from build123d import *

# Parameters (mm, degrees)
BENCH_FRAME_EXTRUDE_DEPTH    = 3
CURVED_PANEL_CLEARANCE_DEPTH = 4
POD_FOOT_CLEARANCE_SKETCH_R  = 1.7
POD_FOOT_THROUGH_HOLES_DEPTH = 4
FOOT_COUNTERBORE_SKETCH_R    = 3.6
FOOT_COUNTERBORES_DEPTH      = 2.9


with BuildPart() as part:
    # Bench Frame Sketch → Bench Frame Extrude (new, symmetric)
    with BuildSketch(Plane.XY):
        Polygon((-70, -98), (118, -98), (118, 98), (-70, 98), (-70, 83), (62, 83), (62, -83), (-70, -83), align=None)
    extrude(amount=BENCH_FRAME_EXTRUDE_DEPTH, both=True)

    # Curved Panel Clearance Sketch → Curved Panel Clearance (cut, symmetric)
    with BuildSketch(Plane.XY):
        with BuildLine():
            Line((-51.777652934, 90.5), (-45.159619167, 90.5))
            ThreePointArc((-45.159619167, 90.5), (-65.5, 0), (-45.159619167, -90.5))
            Line((-45.159619167, -90.5), (-51.777652934, -90.5))
            ThreePointArc((-51.777652934, -90.5), (-71.5, 0), (-51.777652934, 90.5))
        make_face()
    extrude(amount=CURVED_PANEL_CLEARANCE_DEPTH, both=True, mode=Mode.SUBTRACT)

    # Pod Foot Clearance Sketch → Pod Foot Through Holes (cut, symmetric)
    with BuildSketch(Plane.XY):
        with Locations((-14, -87.5)):
            Circle(POD_FOOT_CLEARANCE_SKETCH_R)
        with Locations((16, -87.5)):
            Circle(POD_FOOT_CLEARANCE_SKETCH_R)
        with Locations((-14, 87.5)):
            Circle(POD_FOOT_CLEARANCE_SKETCH_R)
        with Locations((16, 87.5)):
            Circle(POD_FOOT_CLEARANCE_SKETCH_R)
        with Locations((40.25, 87.5)):
            Circle(POD_FOOT_CLEARANCE_SKETCH_R)
        with Locations((-40.5, 87.5)):
            Circle(POD_FOOT_CLEARANCE_SKETCH_R)
        with Locations((86, 22)):
            Circle(POD_FOOT_CLEARANCE_SKETCH_R)
        with Locations((86, 46)):
            Circle(POD_FOOT_CLEARANCE_SKETCH_R)
        with Locations((90, 30)):
            Circle(POD_FOOT_CLEARANCE_SKETCH_R)
        with Locations((97, 26)):
            Circle(POD_FOOT_CLEARANCE_SKETCH_R)
        with Locations((100, 33.5)):
            Circle(POD_FOOT_CLEARANCE_SKETCH_R)
    extrude(amount=POD_FOOT_THROUGH_HOLES_DEPTH, both=True, mode=Mode.SUBTRACT)

    # Foot Counterbore Sketch → Foot Counterbores (cut)
    with BuildSketch(Plane.XY.offset(-3)):
        with Locations((-14, -87.5)):
            Circle(FOOT_COUNTERBORE_SKETCH_R)
        with Locations((16, -87.5)):
            Circle(FOOT_COUNTERBORE_SKETCH_R)
        with Locations((-14, 87.5)):
            Circle(FOOT_COUNTERBORE_SKETCH_R)
        with Locations((16, 87.5)):
            Circle(FOOT_COUNTERBORE_SKETCH_R)
        with Locations((40.25, 87.5)):
            Circle(FOOT_COUNTERBORE_SKETCH_R)
        with Locations((-40.5, 87.5)):
            Circle(FOOT_COUNTERBORE_SKETCH_R)
        with Locations((86, 22)):
            Circle(FOOT_COUNTERBORE_SKETCH_R)
        with Locations((86, 46)):
            Circle(FOOT_COUNTERBORE_SKETCH_R)
        with Locations((90, 30)):
            Circle(FOOT_COUNTERBORE_SKETCH_R)
        with Locations((97, 26)):
            Circle(FOOT_COUNTERBORE_SKETCH_R)
        with Locations((100, 33.5)):
            Circle(FOOT_COUNTERBORE_SKETCH_R)
    extrude(amount=FOOT_COUNTERBORES_DEPTH, mode=Mode.SUBTRACT)


solid = part.part
Geometry: final body of the model. Coordinates: model frame, mm. A direction names the side the tool comes from. Give positions to 0.01 mm unless a question says otherwise; leave off trailing zeros. Write each loop counter-clockwise with the first axis right and the second up, starting at its lowest first coordinate (ties: lowest second). Pieces come first, ordered by that corner, then holes. Notation, with made-up numbers: M -15,-18 L 10,-18 A17 ccw 10,10 Z; hole C 32,-37.75 d5. An arc over 180 degrees is marked long. Answer in a Markdown table with one row per item. Add a question column.
(1) First-contact query: pin 1 (3.5 mm diameter, centred on x = 14.5, y = 88, fed in from -Z). Flat tip, straight axial feed; report the tip coordinate or a pass-through.
(2) Section C-C on y = -1.5. Return loops of the section in (x, z), and give its area (3 significant figures).
(3) Section A-A on x = -7. Return loops of the section in (y, z), and give its area (3 significant figures).
(4) Mould query, pull axis Y, two halves, no side actions, for faces 1 (the cylindrical face through (87.661, 18.806, -1.57)), 2 (the flat face through (25, 98, 0)), 3 (the flat face through (64, 1, 3)). Classes: +Y half, -Y half, draft (parallel to the pull), parting line (faces both ways), or undercut.
(5) Reachability of faces 4 (the cylindrical face through (-53.42, -86.82, 0.04)), 5 (the flat face through (-63, 83, 0)), 6 (the cylindrical face through (-40.97, 91.07, -1.57)), 7 (the flat face through (64, 1, -3)), 8 (the flat face through (-70, -90, 0)) from +Z, -Z, +X, -X, +Y, -Y: full face, straight path, thin tool, end or side. Return the list, or none.
(6) Section B-B on z = 1.65. State how many separate pieces and enclosed holes the cut face has, and give its area (3 significant figures).
(7) Ray query, line 1 (Y direction, x = 40.25, z = 1.45); line 2 (Y direction, x = 16, z = 2.2); line 3 (Y direction, x = 40.25, z = -1.3). Return the intervals inside material, ascending.
Result set:
| question | item | result |
|---|---|---|
| 1 | pin 1 | stops at z = -0.1 |
| 2 | outline | M 62,-3 L 118,-3 L 118,3 L 62,3 Z |
| 2 | area | 336 mm^2 |
| 3 | outline | M -98,-3 L -83,-3 L -83,3 L -98,3 Z; M 83,-3 L 98,-3 L 98,3 L 83,3 Z |
| 3 | area | 180 mm^2 |
| 4 | face 1 | undercut |
| 4 | face 2 | +Y half |
| 4 | face 3 | draft |
| 5 | face 4 | +Z, -Z |
| 5 | face 5 | +Z, -Z, -X |
| 5 | face 6 | -Z |
| 5 | face 7 | -Z, +X, -X, +Y, -Y |
| 5 | face 8 | +Z, -Z, -X, +Y, -Y |
| 6 | separate pieces | 1 |
| 6 | enclosed holes | 11 |
| 6 | area | 14,700 mm^2 |
| 7 | line 1 | y = -98 to -83, 83 to 85.8, 89.2 to 98 |
| 7 | line 2 | y = -98 to -89.2, -85.8 to -83, 83 to 85.8, 89.2 to 98 |
| 7 | line 3 | y = -98 to -83, 83 to 83.9, 91.1 to 98 |
